Source: CAD feature listing. Evaluate the final solid. Frame: model axes, mm. Face numbers are marked on the shaded views. A direction names the side the tool comes from. Give positions to 0.01 mm unless a question says otherwise; leave off trailing zeros. Order: outer loops, then holes, each group sorted by start corner. A loop starts at its lowest first (then second) coordinate and runs counter-clockwise, first axis right, second up.
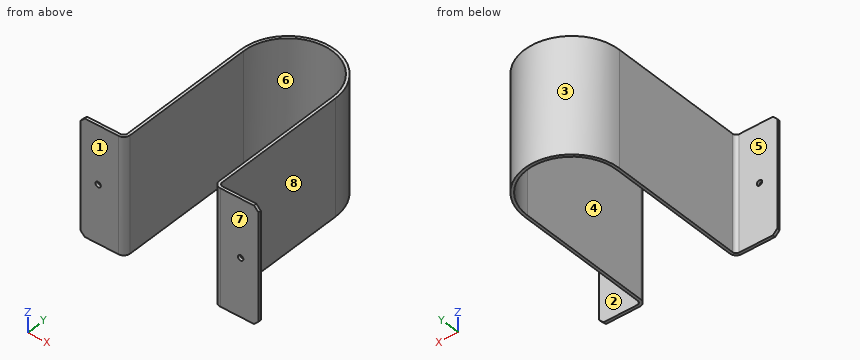
```python
from build123d import *

# Parameters (mm, degrees)
BASE_FLANGE1_DEPTH = 65
SKETCH6_R          = 3
CUT_EXTRUDE1_DEPTH = 10
CHAMFER1_SIZE      = 5


# Sheet-metal steps are written as plain solids
with BuildPart() as part:
    # Sketch1 → Base-Flange1 (new, symmetric)
    with BuildSketch(Plane.XY):
        with BuildLine():
            Line((-100, 0), (-57.175, 0))
            ThreePointArc((-57.175, 0), (-52.101508845, 2.101508845), (-50, 7.175))
            Line((-50, 7.175), (-50, 160))
            ThreePointArc((-50, 160), (0, 210), (50, 160))
            Line((50, 160), (50, 7.175))
            ThreePointArc((50, 7.175), (52.101508845, 2.101508845), (57.175, 0))
            Line((57.175, 0), (100, 0))
            Line((100, 0), (100, 3.175))
            Line((100, 3.175), (57.175, 3.175))
            ThreePointArc((57.175, 3.175), (54.346572875, 4.346572875), (53.175, 7.175))
            Line((53.175, 7.175), (53.175, 160))
            ThreePointArc((53.175, 160), (0, 213.175), (-53.175, 160))
            Line((-53.175, 160), (-53.175, 7.175))
            ThreePointArc((-53.175, 7.175), (-54.346572875, 4.346572875), (-57.175, 3.175))
            Line((-57.175, 3.175), (-100, 3.175))
            Line((-100, 3.175), (-100, 0))
        make_face()
    extrude(amount=BASE_FLANGE1_DEPTH, both=True)

    # Sketch6 → Cut-Extrude1 (cut)
    with BuildSketch(Plane(origin=(0, 3.175, 0), x_dir=(1, 0, 0), z_dir=(0, 1, 0))):
        with Locations(Location((80, 0, 0), (0, 0, 270))):
            Circle(SKETCH6_R)
        with Locations(Location((-80, 0, 0), (0, 0, 270))):
            Circle(SKETCH6_R)
    extrude(amount=-CUT_EXTRUDE1_DEPTH, mode=Mode.SUBTRACT)

    # Chamfer1
    chamfer1_edges = [part.edges().sort_by_distance(p)[0] for p in [
        (-100, 1.5875, -65),
        (100, 1.5875, -65),
        (-100, 1.5875, 65),
        (100, 1.5875, 65),
    ]]
    chamfer(chamfer1_edges, length=CHAMFER1_SIZE)


solid = part.part
```
1) Draft query along X for the marked faces 6, 7 and 8. Return one class per face: +X half, -X half, draft (parallel to the pull), parting line (faces both ways), or undercut.
Report:
face 6: undercut
face 7: draft
face 8: +X half
2) Material intervals for L1, parallel to X at y = 117, z = -49.5 (3 decimals); L2, parallel to X at y = 1, z = 0; L3, parallel to X at y = 2, z = 0, sorted ascending.
Report:
L1: x = -53.175 to -50, 50 to 53.175
L2: x = -100 to -83, -77 to -53.52, 53.52 to 77, 83 to 100
L3: x = -100 to -83, -77 to -52.21, 52.21 to 77, 83 to 100
3) Section query C-C, the plane x = -80. Return the cut outline in (y, z) (3 decimals), and give its area (3 significant figures).
Report:
outline: (0, -65) - (3.175, -65) - (3.175, -3) - (0, -3) - close; (0, 3) - (3.175, 3) - (3.175, 65) - (0, 65) - close
area: 394 mm2
4) Reachability of the marked faces 1, 2, 3, 4 and 5 from +Z, -Z, +X, -X, +Y, -Y: full face, straight path, thin tool, end or side. Return the list, or none.
Report:
face 1: +Z, -Z, +X, -X, -Y
face 2: +Z, -Z, +X, +Y
face 3: +Z, -Z, +Y
face 4: +Z, -Z, -Y
face 5: +Z, -Z, -X, +Y
5) Section query B-B, the plane y = 92. Return the cut outline in (x, z) (3 decimals).
Report:
outline: (-53.175, -65) - (-50, -65) - (-50, 65) - (-53.175, 65) - close; (50, -65) - (53.175, -65) - (53.175, 65) - (50, 65) - close
6) Section query D-D, the plane z = -34. Return the cut outline in (x, y) (3 decimals).
Report:
outline: (-100, 0) - (-57.175, 0) arc R7.175 ccw to (-50, 7.175) - (-50, 160) arc R50 cw to (50, 160) - (50, 7.175) arc R7.175 ccw to (57.175, 0) - (100, 0) - (100, 3.175) - (57.175, 3.175) arc R4 cw to (53.175, 7.175) - (53.175, 160) arc R53.175 ccw to (-53.175, 160) - (-53.175, 7.175) arc R4 cw to (-57.175, 3.175) - (-100, 3.175) - close
7) Section query A-A, the plane z = 0. Return the cut outline in (x, y) (3 decimals).
Report:
outline: (-100, 0) - (-83, 0) - (-83, 3.175) - (-100, 3.175) - close; (-77, 0) - (-57.175, 0) arc R7.175 ccw to (-50, 7.175) - (-50, 160) arc R50 cw to (50, 160) - (50, 7.175) arc R7.175 ccw to (57.175, 0) - (77, 0) - (77, 3.175) - (57.175, 3.175) arc R4 cw to (53.175, 7.175) - (53.175, 160) arc R53.175 ccw to (-53.175, 160) - (-53.175, 7.175) arc R4 cw to (-57.175, 3.175) - (-77, 3.175) - close; (83, 0) - (100, 0) - (100, 3.175) - (83, 3.175) - close
8) Pin query (flat end, axial travel): pin 1 (5 mm diameter, centred on y = 142.5, z = 0.5, fed in from -X) (3 decimals); pin 2 (3.5 mm diameter, centred on x = -80, z = 0, fed in from +Y); pin 3 (1 mm diameter, centred on x = 6, z = -9, fed in from -Y); pin 4 (5 mm diameter, centred on x = -35, z = 44.5, fed in from +Y). Return the tip coordinate at first contact, or that it passes through.
Report:
pin 1: stops at x = -53.175
pin 2: passes through
pin 3: stops at y = 209.58
pin 4: stops at y = 202.09
